Check sheet for the modelled part. Datum: model origin and axes. Units: mm. Give positions to 0.01 mm unless a question says otherwise; leave off trailing zeros. Write each loop counter-clockwise with the first axis right and the second up, starting at its lowest first coordinate (ties: lowest second). Pieces come first, ordered by that corner, then holes. Notation, with made-up numbers: (56, 44.25) - (65, 44.25) arc R31 cw to (65, 75.25) - close; hole circle Ø6 at (14.5, -16). An arc over 180 degrees is marked (long way). Return JSON: item names as keys, results as strings. Group by question number.
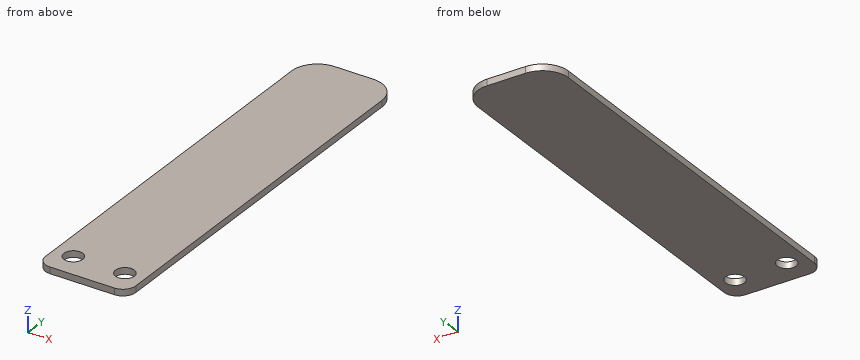
Autodesk Inventor part; units mm, degrees
ref_plane "YZ Plane" through (0, 0, 0) normal (1, 0, 0) x (0, 1, 0)
ref_plane "XZ Plane" through (0, 0, 0) normal (0, 1, 0) x (-1, 0, 0)
ref_plane "XY Plane" through (0, 0, 0) normal (0, 0, 1) x (1, 0, 0)
sketch "Sketch1" plane through (0, 0, 0) normal (0, 0, 1) x (1, 0, 0)
  circle A0 centre (0, 0) radius 2.3241
  line L0 (0, 0) -> (12.7, 0)
  line L1 (0, 0) -> (-12.7, 0)
  circle A1 centre (-12.7, 0) radius 2.3241
  circle A2 centre (12.7, 0) radius 2.3241
  line L2 (-19.05, -6.35) -> (19.05, -6.35)
  line L3 (19.05, -6.35) -> (19.05, 6.35)
  line L4 (19.05, 6.35) -> (-19.05, 6.35)
  line L5 (-19.05, 6.35) -> (-19.05, -6.35)
  line L6 (-19.05, -6.35) -> (19.05, 6.35) construction
  line L7 (19.05, -6.35) -> (-19.05, 6.35) construction
  line L8 (-19.05, 6.35) -> (19.05, 6.35)
  line L9 (19.05, 6.35) -> (19.05, 95.25)
  line L10 (19.05, 95.25) -> (-19.05, 95.25)
  line L11 (-19.05, 95.25) -> (-19.05, 6.35)
  line L12 (-19.05, -6.35) -> (-17.4625, -6.35)
  line L13 (19.05, -6.35) -> (17.4625, -6.35)
  line L14 (-17.4625, -6.35) -> (-17.4625, 95.25)
  line L15 (17.4625, -6.35) -> (17.4625, 95.25)
  dimension "d0" = 4.6482
  dimension "d1" = 12.7
  dimension "d2" = 12.7
  dimension "d3" = 4.6482
  dimension "d4" = 4.6482
  dimension "d5" = 38.1
  dimension "d6" = 12.7
  dimension "d7" = 88.9
  dimension "d8" = 38.1
  dimension "d11" = 1.5875
  dimension "d12" = 1.5875
extrude "Extrusion1" add sketch "Sketch1" along normal blind 1.5875
extrude "Extrusion2" cut sketch "Sketch1" along normal through all contours L5 L4 L14 L2 | L11 L10 L14 L4 | L15 L4 L3 L2 | L15 L10 L9 L4
fillet "Fillet1" radius 3.175 2 edges at (-17.4625, -6.35, 0.7937) (17.4625, -6.35, 0.7937)
fillet "Fillet2" radius 6.35 2 edges at (-17.4625, 95.25, 0.7937) (17.4625, 95.25, 0.7937)
sketch "Sketch2" plane through (0, 0, 1.5875) normal (0, 0, 1) x (1, 0, 0)
  arc A0 (17.4625, 88.9) -> (11.1125, 95.25) centre (11.1125, 88.9) ccw
  line L0 (11.1125, 95.25) -> (-11.1125, 95.25)
  arc A1 (-11.1125, 95.25) -> (-17.4625, 88.9) centre (-11.1125, 88.9) ccw
  line L1 (-17.4625, 88.9) -> (-17.4625, -3.175)
  arc A2 (-17.4625, -3.175) -> (-14.2875, -6.35) centre (-14.2875, -3.175) ccw
  line L2 (-14.2875, -6.35) -> (14.2875, -6.35)
  arc A3 (14.2875, -6.35) -> (17.4625, -3.175) centre (14.2875, -3.175) ccw
  line L3 (17.4625, -3.175) -> (17.4625, 88.9)
  circle A4 centre (12.7, 0) radius 2.3241
  circle A5 centre (0, 0) radius 2.3241
  circle A6 centre (-12.7, 0) radius 2.3241
  line L4 (-17.4625, 10.0615) -> (-4.7625, 10.0615)
  line L5 (-4.7625, -6.35) -> (-31.8174, -6.35)
  line L6 (-31.8174, -6.35) -> (-31.8174, 101.6265)
  line L7 (-31.8174, 101.6265) -> (-4.7625, 101.6265)
  line L8 (-4.7625, 101.6265) -> (-4.7625, -6.35)
  point P0 (-4.7625, 95.25)
  dimension "d17" = 12.7
extrude "Extrusion3" cut sketch "Sketch2" against normal blind 25.4 contours L8 L4 L1 A1 L0 | L8 L2 A2 L1 L4
fillet "Fillet3" radius 3.175 1 edges at (-4.7625, -6.35, 0.7937)
fillet "Fillet4" radius 6.35 1 edges at (-4.7625, 95.25, 0.7937)
properties part number "American Flag Replacement"
Item 1: Material ranges on line 1 along Y through (x, z) = (-1.5, 0.25); line 2 along Y through (x, z) = (0, 0.9); line 3 along Y through (x, z) = (-3.5, 0.95), recorded low to high. Write a range as from..to.
Item 2: Section check A-A on y = 0. Record the cut outline in (x, z), plus the area to 3 significant figures.
Item 3: Section check C-C on x = 12.7. Record the cut outline in (y, z).
Item 4: Section check B-B on z = 0.85. Count the separate pieces of the cut face and the enclosed holes in it, plus the area to 3 significant figures.
Reply:
{
 "1": {"line 1": "-6.35..-1.78, 1.78..94.45", "line 2": "-6.35..-2.32, 2.32..95.05", "line 3": "-5.71..92.7"},
 "2": {"outline": "(-4.76, 0) - (-2.32, 0) - (-2.32, 1.59) - (-4.76, 1.59) - close; (2.32, 0) - (10.38, 0) - (10.38, 1.59) - (2.32, 1.59) - close; (15.02, 0) - (17.46, 0) - (17.46, 1.59) - (15.02, 1.59) - close", "area": "20.5 mm²"},
 "3": {"outline": "(-6.35, 0) - (-2.32, 0) - (-2.32, 1.59) - (-6.35, 1.59) - close; (2.32, 0) - (95.05, 0) - (95.05, 1.59) - (2.32, 1.59) - close"},
 "4": {"separate pieces": "1", "enclosed holes": "2", "area": "2,200 mm²"}
}
